```python
from build123d import *

# Parameters (mm, degrees)
SKETCH1_R               = 7
BOSS_EXTRUDE1_DEPTH     = 50
SKETCH2_W               = 0.776080751
SKETCH2_H               = 12.3835138
CUT_EXTRUDE1_DEPTH      = 100
CUT_EXTRUDE2_DEPTH      = 40
CUT_EXTRUDE2_DEPTH_BACK = 40
SKETCH3_R               = 3


with BuildPart() as part:
    # Sketch1 → Boss-Extrude1 (new body)
    with BuildSketch(Plane(origin=(0, 0, 0), x_dir=(1, 0, 0), z_dir=(0, 1, 0))):
        with Locations(Location((0, 0, 0), (0, 0, 270))):
            Circle(SKETCH1_R)
    extrude(amount=BOSS_EXTRUDE1_DEPTH)

    # Sketch2 → Cut-Extrude1 (cut)
    with BuildSketch(Plane(origin=(0, 50, 0), x_dir=(1, 0, 0), z_dir=(0, 1, 0))):
        with Locations((-0.111959624, 1.211880607)):
            Rectangle(SKETCH2_W, SKETCH2_H)
    extrude(amount=-CUT_EXTRUDE1_DEPTH, mode=Mode.SUBTRACT)

    # Sketch3 → Cut-Extrude2 (cut, two sides: drawn at the far end of the back side and taken through both)
    with BuildSketch(Plane(origin=(0, 0, 0), x_dir=(0, 0, -1), z_dir=(1, 0, 0)).offset(-CUT_EXTRUDE2_DEPTH_BACK)):
        with Locations(Location((-0.002723223, 15, 0), (0, 0, 180))):
            Circle(SKETCH3_R)
        with Locations(Location((-0.002723223, 45.179912014, 0), (0, 0, 180))):
            Circle(SKETCH3_R)
    extrude(amount=CUT_EXTRUDE2_DEPTH + CUT_EXTRUDE2_DEPTH_BACK, mode=Mode.SUBTRACT)


solid = part.part
```
Design review of the part built by this model. Coordinates are the model's own, in mm. A direction names the side the tool comes from. Round coordinates to 2 decimals unless told otherwise and drop trailing zeros. Write each loop counter-clockwise with the first axis right and the second up, starting at its lowest first coordinate (ties: lowest second). Pieces come first, ordered by that corner, then holes.
Item 1: Clearance check with flat-ended pins moving along their axes: pin 1 Ø3 at (y, z) = (33.5, -3.5) entering from +X; pin 2 Ø1 at (x, y) = (-1.5, 12) entering from +Z; pin 3 Ø3 at (x, y) = (-1.5, 41) entering from -Z. State where each tip first meets the part, or that it passes through.
Item 2: We need section A-A on z = 0. Write out the cut boundary in (x, y).
Item 3: We need section C-C on x = 3. Write out the cut boundary in (y, z), and give its area (3 significant figures).
Item 4: The part is to be moulded in two halves that separate along Y. For faces 1 (the flat face through (-1, 0, 0)), 2 (the flat face through (0.276, 25, -1)), 3 (the cylindrical face through (-3.798, 16.149, 2.774)), say which applies: +Y half, -Y half, draft (parallel to the pull), parting line (faces both ways), or undercut.
Item 5: We need section D-D on y = 23.5. Write out the cut boundary in (x, z), and give its area (3 significant figures).
Item 6: We need section B-B on z = -3.5. Write out the cut boundary in (x, y).
Item 7: For probe 1 along Y at (x, z) = (5.5, -1.75); probe 2 along X at (y, z) = (23, -0.25); probe 3 along Y at (x, z) = (-3, 1.25), list the stretches that pass through material, from the lowest coordinate up.
Item 8: For faces 4 (the flat face through (-0.5, 25, -1)), 5 (the cylindrical face through (3.594, 42.205, -0.388)), list the 3-axis set-ups (+Z, -Z, +X, -X, +Y, -Y) from which the entire face can be reached by the end or side of a thin tool; tool diameter is ignored.
Returned:
1. pin 1: stops at x = 6.71
1. pin 2: stops at z = 6.93
1. pin 3: stops at z = -6.98
2. outline: (-7, 0) - (-0.5, 0) - (-0.5, 12) - (-7, 12) - close; (-7, 18) - (-0.5, 18) - (-0.5, 42.18) - (-7, 42.18) - close; (-7, 48.18) - (-0.5, 48.18) - (-0.5, 50) - (-7, 50) - close; (0.28, 0) - (7, 0) - (7, 12) - (0.28, 12) - close; (0.28, 18) - (7, 18) - (7, 42.18) - (0.28, 42.18) - close; (0.28, 48.18) - (7, 48.18) - (7, 50) - (0.28, 50) - close
3. outline: (0, -6.32) - (50, -6.32) - (50, 6.32) - (0, 6.32) - close; hole circle Ø6 at (15, 0); hole circle Ø6 at (45.18, 0)
3. area: 576 mm2
4. face 1: -Y half
4. face 2: draft
4. face 3: undercut
5. outline: (-0.5, -6.98) - (-0.5, 4.98) - (0.28, 4.98) - (0.28, -6.99) arc R7 ccw (long way) to start
5. area: 145 mm2
6. outline: (-6.06, 0) - (-0.5, 0) - (-0.5, 50) - (-6.06, 50) - close; (0.28, 0) - (6.06, 0) - (6.06, 50) - (0.28, 50) - close
7. probe 1: y = 0 to 12.57, 17.43 to 42.75, 47.61 to 50
7. probe 2: x = -7 to -0.5, 0.28 to 7
7. probe 3: y = 0 to 12.27, 17.73 to 42.45, 47.91 to 50
8. face 4: -Z, +Y, -Y
8. face 5: +X, -X
